The listing builds one solid part. Answer for the finished solid, in the listing's coordinates (mm). A direction names the side the tool comes from. Give positions to 0.01 mm unless a question says otherwise; leave off trailing zeros. Loops run counter-clockwise (first coordinate to the right, second up) from the corner with the lowest first, then second, coordinate; pieces in that order, holes last. Notation, with made-up numbers: M 16.25,72.5 L 37.25,72.5 A21 cw 37.25,96.5 Z; hole C 26.5,20 d3. An arc over 180 degrees is marked long. Return JSON: item names as keys, results as strings.
from build123d import *

# Parameters (mm, degrees)
F0_W     = 40
F0_H     = 40
F1_DEPTH = 40
F3_DEPTH = 10


with BuildPart() as f1:
    # F0 (on Front) → F1 (new body)
    with BuildSketch(Plane.XZ):
        Rectangle(F0_W, F0_H)
    extrude(amount=F1_DEPTH)

    # F2 (on Top) → F3 (join, symmetric)
    with BuildSketch(Plane.XY):
        Polygon((-5, 0), (5, 0), (10, 20), (-10, 20), align=None)
    extrude(amount=F3_DEPTH, both=True)


solid = f1.part
(1) Determine the mould class of faces 6 (the flat face through (7.465, 9.86, 0.14)), 7 (the flat face through (0, 20, 0)), 8 (the flat face through (-20, -20, 0)), 9 (the flat face through (9, 0, 0)) for opening direction Y: released by +Y, released by -Y, zero draft, split by the parting line, or undercut.
Values follow:
{"face 6": "undercut", "face 7": "released by +Y", "face 8": "zero draft", "face 9": "undercut"}
(2) Straight lines are drawn through the part: line 1 along Z through (x, y) = (-7, 9); line 2 along Y through (x, z) = (-17, -16); line 3 along X through (y, z) = (15, -5.5). For each, find the intervals that lie inside material, in ascending order.
Values follow:
{"line 1": "-10 to 10", "line 2": "-40 to 0", "line 3": "-8.75 to 8.75"}
(3) The part is cut by section C-C (x = 1). Determine the outline of the cut face in (y, z).
Values follow:
{"outline": "M -40,-20 L 0,-20 L 0,-10 L 20,-10 L 20,10 L 0,10 L 0,20 L -40,20 Z"}
(4) Given pin 1 (6 mm diameter, centred on x = 4, y = 4.5, fed in from +Z); pin 2 (16 mm diameter, centred on x = 1.5, y = 6.5, fed in from -Z), each flat-ended and moving along its own axis, determine where each tip first touches the part or whether it passes through.
Values follow:
{"pin 1": "z = 10", "pin 2": "z = -20"}
(5) A tool of negligible diameter and unlimited length cuts with its end or side. For faces 1 (the flat face through (0, -40, 0)), 2 (the flat face through (-7.535, 10.14, 0.14)), 3 (the flat face through (0, 12, -10)), 4 (the flat face through (0, -20, -20)), 5 (the flat face through (0, 12, 10)), from which of +Z, -Z, +X, -X, +Y, -Y can it reach the whole face along a straight path? Write none if from no direction.
Values follow:
{"face 1": "+Z, -Z, +X, -X, -Y", "face 2": "+Z, -Z, -X", "face 3": "-Z, +X, -X, +Y", "face 4": "-Z, +X, -X, +Y, -Y", "face 5": "+Z, +X, -X, +Y"}
(6) The part is cut by section A-A (x = 9). Determine the outline of the cut face in (y, z).
Values follow:
{"outline": "M -40,-20 L 0,-20 L 0,20 L -40,20 Z; M 16,-10 L 20,-10 L 20,10 L 16,10 Z"}
(7) The part is cut by section D-D (z = -12). Determine the outline of the cut face in (x, y).
Values follow:
{"outline": "M -20,-40 L 20,-40 L 20,0 L -20,0 Z"}
(8) The part is cut by section B-B (z = -5). Determine the outline of the cut face in (x, y).
Values follow:
{"outline": "M -20,-40 L 20,-40 L 20,0 L 5,0 L 10,20 L -10,20 L -5,0 L -20,0 Z"}
